```python
from build123d import *

# Parameters (mm, degrees)
EXTRUDE_1_DEPTH        = 7
EXTRUDE_1_DEPTH_BACK   = 7
SKETCH_1_W             = 15
SKETCH_1_H             = 34.3
SKETCH_1_R             = 1.5
EXTRUDE_1_2_DEPTH      = 7
EXTRUDE_1_2_DEPTH_BACK = 7
SKETCH_2_W             = 9.2
SKETCH_2_H             = 6.7
CUT_EXTRUDE_1_DEPTH    = 62
SKETCH_3_W             = 24
SKETCH_3_H             = 23.2
EXTRUDE_2_DEPTH        = 12
SKETCH_4_R             = 2.5
CUT_EXTRUDE_2_DEPTH    = 90
FILLET_1_R             = 2
CHAMFER_1_SIZE         = 5
CHAMFER_2_SIZE         = 5
FILLET_2_R             = 2


with BuildPart() as part:
    # Sketch 1 → Extrude 1 (new, two sides: drawn at the far end of the back side and taken through both)
    with BuildSketch(Plane.XY.offset(-EXTRUDE_1_DEPTH_BACK)):
        with Locations((30, 0)):
            Rectangle(SKETCH_1_W, SKETCH_1_H)
        with Locations((30, 10)):
            Circle(SKETCH_1_R, mode=Mode.SUBTRACT)
        with Locations(Location((30, -10, 0), (0, 0, 180))):
            Circle(SKETCH_1_R, mode=Mode.SUBTRACT)
    extrude(amount=EXTRUDE_1_DEPTH + EXTRUDE_1_DEPTH_BACK)


with BuildPart() as body_2:
    # Sketch 1 → Extrude 1 2 (new, two sides: drawn at the far end of the back side and taken through both)
    with BuildSketch(Plane.XY.offset(-EXTRUDE_1_2_DEPTH_BACK)):
        with Locations((-30, 0)):
            Rectangle(SKETCH_1_W, SKETCH_1_H)
        with Locations((-30, -10)):
            Circle(SKETCH_1_R, mode=Mode.SUBTRACT)
        with Locations(Location((-30, 10, 0), (0, 0, 180))):
            Circle(SKETCH_1_R, mode=Mode.SUBTRACT)
    extrude(amount=EXTRUDE_1_2_DEPTH + EXTRUDE_1_2_DEPTH_BACK)


with BuildPart() as cut_extrude_1_tool:
    # Sketch 2 → Cut-Extrude 1 (new body)
    with BuildSketch(Plane(origin=(0, 17.15, 0), x_dir=(1, 0, 0), z_dir=(0, 1, 0))):
        with Locations((30, 0)):
            Rectangle(SKETCH_2_W, SKETCH_2_H)
        with Locations((-30, 0)):
            Rectangle(SKETCH_2_W, SKETCH_2_H)
    extrude(amount=-CUT_EXTRUDE_1_DEPTH)


with BuildPart() as part_1:
    add(part.part)

    # Cut-Extrude 1: cut by cut_extrude_1_tool
    add(cut_extrude_1_tool.part, mode=Mode.SUBTRACT)



with BuildPart() as body_2_1:
    add(body_2.part)

    # Cut-Extrude 1: cut by cut_extrude_1_tool
    add(cut_extrude_1_tool.part, mode=Mode.SUBTRACT)


with BuildPart() as part_2:
    add(part_1.part)

    add(body_2_1.part)  # Extrude 2 merges body 2
    # Sketch 3 → Extrude 2 (add)
    with BuildSketch(Plane(origin=(0, 17.15, 0), x_dir=(1, 0, 0), z_dir=(0, 1, 0))):
        Polygon((22.5, 7), (17, 7), (17, 17.5), (-17, 17.5), (-17, 7), (-22.5, 7), (-22.5, -7), (-17, -7), (-17, -17.5), (17, -17.5), (17, -7), (22.5, -7), align=None)
        Rectangle(SKETCH_3_W, SKETCH_3_H, mode=Mode.SUBTRACT)
    extrude(amount=-EXTRUDE_2_DEPTH)

    # Sketch 4 → Cut-Extrude 2 (cut)
    with BuildSketch(Plane.XY.offset(17.5)):
        with Locations((0, 11.15)):
            Circle(SKETCH_4_R)
    extrude(amount=-CUT_EXTRUDE_2_DEPTH, mode=Mode.SUBTRACT)

    # Fillet 1
    fillet_1_edges = [part_2.edges().sort_by_distance(p)[0] for p in [
        (-37.5, 0, -7),
        (-37.5, 0, 7),
        (37.5, 0, 7),
        (37.5, 0, -7),
    ]]
    fillet(fillet_1_edges, radius=FILLET_1_R)

    # Chamfer 1
    chamfer_1_edges = [part_2.edges().sort_by_distance(p)[0] for p in [
        (22.5, 5.15, 0),
        (-22.5, 5.15, 0),
    ]]
    chamfer(chamfer_1_edges, length=CHAMFER_1_SIZE)

    # Chamfer 2
    # the kernel refuses this chamfer: 5 mm, written as the material it adds along each edge
    with BuildSketch(Plane(origin=(17, 17.15, -7), x_dir=(0.9996219169112968, 0, 0.027495876610586147), z_dir=(0, -1, 0))) as chamfer_2_piece_1_section:
        Polygon((CHAMFER_2_SIZE * 0.999621916911, -CHAMFER_2_SIZE * 0.0274958766106), (-CHAMFER_2_SIZE * 0.0274958766106, -CHAMFER_2_SIZE * 0.999621916911), (0, 0), align=None)
    chamfer_2_piece_1 = extrude(amount=12, mode=Mode.PRIVATE)
    chamfer_2_piece_1 = split(chamfer_2_piece_1, bisect_by=Plane(origin=(15.061953737, 7.588046263, -8.643148294), z_dir=(0.7071067811865476, 0.7071067811865475, 0)), keep=Keep.TOP, mode=Mode.PRIVATE)
    add(chamfer_2_piece_1)
    with BuildSketch(Plane(origin=(17, 17.15, -7), x_dir=(0.9996219169112968, 0, 0.027495876610586147), z_dir=(0, -1, 0))) as chamfer_2_piece_2_section:
        Polygon((CHAMFER_2_SIZE * 0.999621916911, -CHAMFER_2_SIZE * 0.0274958766106), (-CHAMFER_2_SIZE * 0.0274958766106, -CHAMFER_2_SIZE * 0.999621916911), (0, 0), align=None)
    chamfer_2_piece_2 = extrude(amount=12, mode=Mode.PRIVATE)
    chamfer_2_piece_2 = split(chamfer_2_piece_2, bisect_by=Plane(origin=(17.181894142, 5.468105858, -9.627776216), z_dir=(-0.7071067811865476, -0.7071067811865475, 0)), keep=Keep.TOP, mode=Mode.PRIVATE)
    add(chamfer_2_piece_2)
    with BuildSketch(Plane(origin=(17, 17.15, -7), x_dir=(0.9996219169112968, 0, 0.027495876610586147), z_dir=(0, -1, 0))) as chamfer_2_piece_3_section:
        Polygon((CHAMFER_2_SIZE * 0.999621916911, -CHAMFER_2_SIZE * 0.0274958766106), (-CHAMFER_2_SIZE * 0.0274958766106, -CHAMFER_2_SIZE * 0.999621916911), (0, 0), align=None)
    chamfer_2_piece_3 = extrude(amount=24.85841494, mode=Mode.PRIVATE)
    chamfer_2_piece_3 = split(chamfer_2_piece_3, bisect_by=Plane(origin=(19.269171179, 3.380828821, -8.010149173), z_dir=(0.7071067811865476, 0.7071067811865475, 0)), keep=Keep.TOP, mode=Mode.PRIVATE)
    chamfer_2_piece_3 = split(chamfer_2_piece_3, bisect_by=Plane(origin=(19.858894906, 5.15, -8.010149173), z_dir=(0, -1, 0)), keep=Keep.TOP, mode=Mode.PRIVATE)
    add(chamfer_2_piece_3)
    with BuildSketch(Plane(origin=(-17, 17.15, -7), x_dir=(0.027495876610586313, 0, -0.9996219169112968), z_dir=(0, -1, 0))) as chamfer_2_piece_4_section:
        Polygon((CHAMFER_2_SIZE * 0.999621916911, -CHAMFER_2_SIZE * 0.0274958766106), (-CHAMFER_2_SIZE * 0.0274958766106, -CHAMFER_2_SIZE * 0.999621916911), (0, 0), align=None)
    chamfer_2_piece_4 = extrude(amount=12, mode=Mode.PRIVATE)
    chamfer_2_piece_4 = split(chamfer_2_piece_4, bisect_by=Plane(origin=(-15.061953737, 7.588046263, -8.643148294), z_dir=(-0.7071067811865475, 0.7071067811865476, 0)), keep=Keep.TOP, mode=Mode.PRIVATE)
    add(chamfer_2_piece_4)
    with BuildSketch(Plane(origin=(-17, 17.15, -7), x_dir=(0.027495876610586313, 0, -0.9996219169112968), z_dir=(0, -1, 0))) as chamfer_2_piece_5_section:
        Polygon((CHAMFER_2_SIZE * 0.999621916911, -CHAMFER_2_SIZE * 0.0274958766106), (-CHAMFER_2_SIZE * 0.0274958766106, -CHAMFER_2_SIZE * 0.999621916911), (0, 0), align=None)
    chamfer_2_piece_5 = extrude(amount=24.85841494, mode=Mode.PRIVATE)
    chamfer_2_piece_5 = split(chamfer_2_piece_5, bisect_by=Plane(origin=(-19.858894906, 5.15, -8.010149173), z_dir=(0, -1, 0)), keep=Keep.TOP, mode=Mode.PRIVATE)
    chamfer_2_piece_5 = split(chamfer_2_piece_5, bisect_by=Plane(origin=(-19.269171179, 3.380828821, -8.010149173), z_dir=(-0.7071067811865475, 0.7071067811865476, 0)), keep=Keep.TOP, mode=Mode.PRIVATE)
    add(chamfer_2_piece_5)
    with BuildSketch(Plane(origin=(-17, 17.15, -7), x_dir=(0.027495876610586313, 0, -0.9996219169112968), z_dir=(0, -1, 0))) as chamfer_2_piece_6_section:
        Polygon((CHAMFER_2_SIZE * 0.999621916911, -CHAMFER_2_SIZE * 0.0274958766106), (-CHAMFER_2_SIZE * 0.0274958766106, -CHAMFER_2_SIZE * 0.999621916911), (0, 0), align=None)
    chamfer_2_piece_6 = extrude(amount=12, mode=Mode.PRIVATE)
    chamfer_2_piece_6 = split(chamfer_2_piece_6, bisect_by=Plane(origin=(-17.181894142, 5.468105858, -9.627776216), z_dir=(0.7071067811865475, -0.7071067811865476, 0)), keep=Keep.TOP, mode=Mode.PRIVATE)
    add(chamfer_2_piece_6)
    with BuildSketch(Plane(origin=(17, 17.15, 7), x_dir=(0.9996219169112968, 0, -0.027495876610586147), z_dir=(0, -1, 0))) as chamfer_2_piece_7_section:
        Polygon((CHAMFER_2_SIZE * 0.999621916911, CHAMFER_2_SIZE * 0.0274958766106), (-CHAMFER_2_SIZE * 0.0274958766106, CHAMFER_2_SIZE * 0.999621916911), (0, 0), align=None)
    chamfer_2_piece_7 = extrude(amount=12, mode=Mode.PRIVATE)
    chamfer_2_piece_7 = split(chamfer_2_piece_7, bisect_by=Plane(origin=(15.061953737, 7.588046263, 8.643148294), z_dir=(0.7071067811865476, 0.7071067811865475, 0)), keep=Keep.TOP, mode=Mode.PRIVATE)
    add(chamfer_2_piece_7)
    with BuildSketch(Plane(origin=(17, 17.15, 7), x_dir=(0.9996219169112968, 0, -0.027495876610586147), z_dir=(0, -1, 0))) as chamfer_2_piece_8_section:
        Polygon((CHAMFER_2_SIZE * 0.999621916911, CHAMFER_2_SIZE * 0.0274958766106), (-CHAMFER_2_SIZE * 0.0274958766106, CHAMFER_2_SIZE * 0.999621916911), (0, 0), align=None)
    chamfer_2_piece_8 = extrude(amount=12, mode=Mode.PRIVATE)
    chamfer_2_piece_8 = split(chamfer_2_piece_8, bisect_by=Plane(origin=(17.181894142, 5.468105858, 9.627776216), z_dir=(-0.7071067811865476, -0.7071067811865475, 0)), keep=Keep.TOP, mode=Mode.PRIVATE)
    add(chamfer_2_piece_8)
    with BuildSketch(Plane(origin=(17, 17.15, 7), x_dir=(0.9996219169112968, 0, -0.027495876610586147), z_dir=(0, -1, 0))) as chamfer_2_piece_9_section:
        Polygon((CHAMFER_2_SIZE * 0.999621916911, CHAMFER_2_SIZE * 0.0274958766106), (-CHAMFER_2_SIZE * 0.0274958766106, CHAMFER_2_SIZE * 0.999621916911), (0, 0), align=None)
    chamfer_2_piece_9 = extrude(amount=24.85841494, mode=Mode.PRIVATE)
    chamfer_2_piece_9 = split(chamfer_2_piece_9, bisect_by=Plane(origin=(19.269171179, 3.380828821, 8.010149173), z_dir=(0.7071067811865476, 0.7071067811865475, 0)), keep=Keep.TOP, mode=Mode.PRIVATE)
    chamfer_2_piece_9 = split(chamfer_2_piece_9, bisect_by=Plane(origin=(19.858894906, 5.15, 8.010149173), z_dir=(0, -1, 0)), keep=Keep.TOP, mode=Mode.PRIVATE)
    add(chamfer_2_piece_9)
    with BuildSketch(Plane(origin=(-17, 17.15, 7), x_dir=(0.027495876610586313, 0, 0.9996219169112968), z_dir=(0, -1, 0))) as chamfer_2_piece_10_section:
        Polygon((CHAMFER_2_SIZE * 0.999621916911, CHAMFER_2_SIZE * 0.0274958766106), (-CHAMFER_2_SIZE * 0.0274958766106, CHAMFER_2_SIZE * 0.999621916911), (0, 0), align=None)
    chamfer_2_piece_10 = extrude(amount=12, mode=Mode.PRIVATE)
    chamfer_2_piece_10 = split(chamfer_2_piece_10, bisect_by=Plane(origin=(-15.061953737, 7.588046263, 8.643148294), z_dir=(-0.7071067811865475, 0.7071067811865476, 0)), keep=Keep.TOP, mode=Mode.PRIVATE)
    add(chamfer_2_piece_10)
    with BuildSketch(Plane(origin=(-17, 17.15, 7), x_dir=(0.027495876610586313, 0, 0.9996219169112968), z_dir=(0, -1, 0))) as chamfer_2_piece_11_section:
        Polygon((CHAMFER_2_SIZE * 0.999621916911, CHAMFER_2_SIZE * 0.0274958766106), (-CHAMFER_2_SIZE * 0.0274958766106, CHAMFER_2_SIZE * 0.999621916911), (0, 0), align=None)
    chamfer_2_piece_11 = extrude(amount=24.85841494, mode=Mode.PRIVATE)
    chamfer_2_piece_11 = split(chamfer_2_piece_11, bisect_by=Plane(origin=(-19.858894906, 5.15, 8.010149173), z_dir=(0, -1, 0)), keep=Keep.TOP, mode=Mode.PRIVATE)
    chamfer_2_piece_11 = split(chamfer_2_piece_11, bisect_by=Plane(origin=(-19.269171179, 3.380828821, 8.010149173), z_dir=(-0.7071067811865475, 0.7071067811865476, 0)), keep=Keep.TOP, mode=Mode.PRIVATE)
    add(chamfer_2_piece_11)
    with BuildSketch(Plane(origin=(-17, 17.15, 7), x_dir=(0.027495876610586313, 0, 0.9996219169112968), z_dir=(0, -1, 0))) as chamfer_2_piece_12_section:
        Polygon((CHAMFER_2_SIZE * 0.999621916911, CHAMFER_2_SIZE * 0.0274958766106), (-CHAMFER_2_SIZE * 0.0274958766106, CHAMFER_2_SIZE * 0.999621916911), (0, 0), align=None)
    chamfer_2_piece_12 = extrude(amount=12, mode=Mode.PRIVATE)
    chamfer_2_piece_12 = split(chamfer_2_piece_12, bisect_by=Plane(origin=(-17.181894142, 5.468105858, 9.627776216), z_dir=(0.7071067811865475, -0.7071067811865476, 0)), keep=Keep.TOP, mode=Mode.PRIVATE)
    add(chamfer_2_piece_12)

    # Fillet 2
    fillet_2_edges = [part_2.edges().sort_by_distance(p)[0] for p in [
        (12, 11.15, -11.6),
        (17, 11.15, 17.5),
        (-17, 11.15, 17.5),
        (-17, 11.15, -17.5),
        (17, 11.15, -17.5),
        (12, 11.15, 11.6),
        (-12, 11.15, 11.6),
        (-12, 11.15, -11.6),
    ]]
    fillet(fillet_2_edges, radius=FILLET_2_R)


solid = part_2.part
```
Source: CAD feature listing. Evaluate the final solid. Frame: model axes, mm. A direction names the side the tool comes from. Coordinates: 2 decimals unless noted, no trailing zeros. Loops run counter-clockwise (first coordinate to the right, second up) from the corner with the lowest first, then second, coordinate; pieces in that order, holes last. Notation, with made-up numbers: (69.5, 62.5) - (101.5, 62.5) arc R12 cw to (101.5, 80.5) - close; hole circle Ø4 at (-20.75, 75.25). An arc over 180 degrees is marked (long way). Answer as CSV lines item,"result".
1. Reachability of faces 1 (the flat face through (22.5, -9, 0)), 2 (the flat face through (-17, 11, -14)), 3 (the flat face through (-17, 11, 14)) from +Z, -Z, +X, -X, +Y, -Y: full face, straight path, thin tool, end or side. Return the list, or none.
Established:
face 1,"+Z, -Z, -Y"
face 2,"-Z, -X, +Y, -Y"
face 3,"+Z, -X, +Y, -Y"
2. Section D-D (x = 0). Return loops of the section in (y, z), then the cut area to 3 significant figures.
Established:
outline,"(5.15, -17.5) - (8.65, -17.5) - (8.65, -11.6) - (5.15, -11.6) - close; (5.15, 11.6) - (8.65, 11.6) - (8.65, 17.5) - (5.15, 17.5) - close; (13.65, -17.5) - (17.15, -17.5) - (17.15, -11.6) - (13.65, -11.6) - close; (13.65, 11.6) - (17.15, 11.6) - (17.15, 17.5) - (13.65, 17.5) - close"
area,"82.6 mm2"
3. Section B-B (x = 30). Return loops of the section in (y, z).
Established:
outline,"(-17.15, -7) - (-11.5, -7) - (-11.5, -3.35) - (-17.15, -3.35) - close; (-17.15, 3.35) - (-11.5, 3.35) - (-11.5, 7) - (-17.15, 7) - close; (-8.5, -7) - (8.5, -7) - (8.5, -3.35) - (-8.5, -3.35) - close; (-8.5, 3.35) - (8.5, 3.35) - (8.5, 7) - (-8.5, 7) - close; (11.5, -7) - (17.15, -7) - (17.15, -3.35) - (11.5, -3.35) - close; (11.5, 3.35) - (17.15, 3.35) - (17.15, 7) - (11.5, 7) - close"
4. Section C-C (z = -0.5). Return loops of the section in (x, y).
Established:
outline,"(-37.5, -17.15) - (-34.6, -17.15) - (-34.6, 17.15) - (-37.5, 17.15) - close; (-25.4, -17.15) - (-22.5, -17.15) - (-22.5, 0.15) - (-17.5, 5.15) - (-12, 5.15) - (-12, 17.15) - (-25.4, 17.15) - close; (12, 5.15) - (17.5, 5.15) - (22.5, 0.15) - (22.5, -17.15) - (25.4, -17.15) - (25.4, 17.15) - (12, 17.15) - close; (34.6, -17.15) - (37.5, -17.15) - (37.5, 17.15) - (34.6, 17.15) - close"
5. Ray query, line 1 (Y direction, x = -30, z = 4.9); line 2 (X direction, y = -10, z = 4.55); line 3 (X direction, y = 11, z = 0.5). Return the intervals inside material, ascending.
Established:
line 1,"y = -17.15 to -11.5, -8.5 to 8.5, 11.5 to 17.15"
line 2,"x = -37.5 to -31.5, -28.5 to -22.5, 22.5 to 28.5, 31.5 to 37.5"
line 3,"x = -37.5 to -34.6, -25.4 to -12, 12 to 25.4, 34.6 to 37.5"
6. Section A-A (y = -3). Return loops of the section in (x, z), then the cut area to 3 significant figures.
Established:
outline,"(-37.5, -5) arc R2 ccw to (-35.5, -7) - (-22.5, -7) - (-22.5, 7) - (-35.5, 7) arc R2 ccw to (-37.5, 5) - close; (22.5, -7) - (35.5, -7) arc R2 ccw to (37.5, -5) - (37.5, 5) arc R2 ccw to (35.5, 7) - (22.5, 7) - close; hole (-34.6, -3.35) - (-25.4, -3.35) - (-25.4, 3.35) - (-34.6, 3.35) - close; hole (25.4, -3.35) - (34.6, -3.35) - (34.6, 3.35) - (25.4, 3.35) - close"
area,"293 mm2"
7. Mould query, pull axis Y, two halves, no side actions, for faces 4 (the cylindrical face through (-0.33, 13.63, -14.51)), 5 (the flat face through (-20.04, 2.61, -0.16)), 6 (the flat face through (17, 11, -14)). Classes: released by +Y, released by -Y, zero draft, split by the parting line, or undercut.
Established:
face 4,"undercut"
face 5,"released by -Y"
face 6,"zero draft"
8. Contact query for flat-ended pins moving along their axis: pin 1 (6 mm diameter, centred on x = 27, y = -4, fed in from +Z); pin 2 (1.5 mm diameter, centred on y = 11, z = -6, fed in from -X); pin 3 (10 mm diameter, centred on x = -29.5, y = -4.5, fed in from -Z). Output: stop coordinate, or through.
Established:
pin 1,"stops at z = 7"
pin 2,"stops at x = -37.48"
pin 3,"stops at z = -7"
